Design review of the part built by this model. Coordinates are the model's own, in mm. A direction names the side the tool comes from. Give positions to 0.01 mm unless a question says otherwise; leave off trailing zeros. Write each loop counter-clockwise with the first axis right and the second up, starting at its lowest first coordinate (ties: lowest second). Pieces come first, ordered by that corner, then holes.
```python
from build123d import *

# Parameters (mm, degrees)
SKETCH1_R            = 9
BOSS_EXTRUDE1_DEPTH  = 12
SKETCH6_W            = 12
SKETCH6_H            = 46
BOSS_EXTRUDE5_DEPTH  = 12
SKETCH7_R            = 8
BOSS_EXTRUDE17_DEPTH = 12


with BuildPart() as part:
    # Sketch1 → Boss-Extrude1 (new body)
    with BuildSketch(Plane.XY):
        with BuildLine():
            Line((-10.505448867, 14.616276684), (53.494551133, 60.616276684))
            ThreePointArc((53.494551133, 60.616276684), (72.212853353, 62.017148304), (82, 46))
            Line((82, 46), (82, -46))
            ThreePointArc((82, -46), (72.212853353, -62.017148304), (53.494551133, -60.616276684))
            Line((53.494551133, -60.616276684), (-10.505448867, -14.616276684))
            ThreePointArc((-10.505448867, -14.616276684), (-18, 0), (-10.505448867, 14.616276684))
        make_face()
        Circle(SKETCH1_R, mode=Mode.SUBTRACT)
        with Locations((64, 46)):
            Circle(SKETCH1_R, mode=Mode.SUBTRACT)
        with Locations((64, -46)):
            Circle(SKETCH1_R, mode=Mode.SUBTRACT)
    extrude(amount=BOSS_EXTRUDE1_DEPTH)

    # Sketch6 → Boss-Extrude5 (add)
    with BuildSketch(Plane(origin=(82, 0, 0), x_dir=(0, 0, -1), z_dir=(1, 0, 0))):
        with Locations((-6, 0)):
            Rectangle(SKETCH6_W, SKETCH6_H)
    extrude(amount=BOSS_EXTRUDE5_DEPTH)

    # Sketch7 → Boss-Extrude17 (add)
    with BuildSketch(Plane.XZ.offset(23)):
        with BuildLine():
            Line((6, 12), (94, 12))
            Line((94, 12), (94, 15.350889359))
            ThreePointArc((94, 15.350889359), (100.88398553, 33.477491841), (83.054187792, 41.097287567))
            Line((83.054187792, 41.097287567), (6, 12))
        make_face()
        with Locations((88, 28)):
            Circle(SKETCH7_R, mode=Mode.SUBTRACT)
    boss_extrude17 = extrude(amount=-BOSS_EXTRUDE17_DEPTH)

    # Mirror2: Boss-Extrude17 across plane
    add(boss_extrude17.mirror(Plane.ZX))


solid = part.part
```
(1) Consider section C-C, the plane x = -4.5. Give the boundary of the cut face in (y, z), then the cut area to 3 significant figures.
Resolved:
outline: (-18.93, 0) - (-7.79, 0) - (-7.79, 12) - (-18.93, 12) - close; (7.79, 0) - (18.93, 0) - (18.93, 12) - (7.79, 12) - close
area: 267 mm2
(2) Tool access review of faces 5 (the face through (68.84, 53.59, 5.92)), 6 (the face through (82, 35, 6)), 7 (the face through (82, -34, 6)): name each direction out of +Z, -Z, +X, -X, +Y, -Y from which nothing blocks a thin tool from reaching the whole face with its end or side.
Resolved:
face 5: +Z, -Z
face 6: +Z, -Z, +X, +Y
face 7: +Z, -Z, +X, -Y
(3) Consider section B-B, the plane x = 88. Give the boundary of the cut face in (y, z).
Resolved:
outline: (-23, 0) - (23, 0) - (23, 20) - (11, 20) - (11, 12) - (-11, 12) - (-11, 20) - (-23, 20) - close; (-23, 36) - (-11, 36) - (-11, 42) - (-23, 42) - close; (11, 36) - (23, 36) - (23, 42) - (11, 42) - close
(4) To check wall thickness, follow L1, parallel to Y at x = 64, z = 7; L2, parallel to Y at x = 72.5, z = 35.5; L3, parallel to Z at x = 85.5, y = 16.5. State the ranges of each line that lie inside material, in increasing order.
Resolved:
L1: y = -64 to -55, -37 to 37, 55 to 64
L2: y = -23 to -11, 11 to 23
L3: z = 0 to 20.4, 35.6 to 41.77
(5) Consider section A-A, the plane z = 5.5. Give the boundary of the cut face in (x, y).
Resolved:
outline: (-10.51, -14.62) - (53.49, -60.62) arc R18 ccw to (82, -46) - (82, -23) - (94, -23) - (94, 23) - (82, 23) - (82, 46) arc R18 ccw to (53.49, 60.62) - (-10.51, 14.62) arc R18 ccw to start; hole circle Ø18 at (0, 0); hole circle Ø18 at (64, -46); hole circle Ø18 at (64, 46)
(6) Mouldability with a two-part tool opening along Y and no side actions: class faces 1 (the face through (21.943, -37.938, 5.916)), 2 (the face through (64, -11, 24)), 3 (the face through (-1.172, 8.923, 5.916)), 4 (the face through (51, 1, 0)) as pulls with the +Y half, pulls with the -Y half, needs draft (parallel to the pull), parting line crosses it, or undercut.
Resolved:
face 1: pulls with the -Y half
face 2: undercut
face 3: undercut
face 4: needs draft
(7) Clearance check with flat-ended pins moving along their axes: P1, Ø21, axis at x = 88, z = 28, coming from the -Y side; P2, Ø9.5, axis at y = -31.5, z = 5, coming from the +X side; P3, Ø15, axis at x = 77, z = 33, coming from the +Y side. State where each tip first meets the part, or that it passes through.
Resolved:
P1: stops at y = -23
P2: stops at x = 82
P3: stops at y = 23
(8) Consider section D-D, the plane y = -6.5. Give the boundary of the cut face in (x, z).
Resolved:
outline: (-16.79, 0) - (-6.22, 0) - (-6.22, 12) - (-16.79, 12) - close; (6.22, 0) - (94, 0) - (94, 12) - (6.22, 12) - close
